For this review, take the finished solid that the model builds, in its own axes (mm). A direction names the side the tool comes from. Coordinates: 2 decimals unless noted, no trailing zeros. Write each loop counter-clockwise with the first axis right and the second up, starting at its lowest first coordinate (ties: lowest second). Pieces come first, ordered by that corner, then holes. Notation, with made-up numbers: (71.5, 4.5) - (116.5, 4.5) arc R17 cw to (116.5, 11.5) - close; hole circle Ø7 at (4, -8.75). An arc over 180 degrees is marked (long way). Use one line per item in the form item = value. Start each with the question number.
1) Mouldability with a two-part tool opening along Y and no side actions: class faces 1 (the flat face through (0, 16.244, 4)), 2 (the flat face through (0, -16.244, 4)), 3 (the flat face through (0, -18.2, 2)), 4 (the flat face through (-5, 21, 2)) as pulls with the +Y half, pulls with the -Y half, needs draft (parallel to the pull), parting line crosses it, or undercut.
2) We need section B-B (y = 15). Give the boundary of the cut face in (x, z).
3) Insertion check: P1, Ø1.5, axis at x = -3, y = 15, coming from the +Z side; P2, Ø3, axis at y = 23.5, z = 4.5, coming from the +X side; P3, Ø1, axis at x = -13, z = 4.5, coming from the +Y side. Each pin has a flat end and moves straight along its axis. Give the tip position at first contact, or say it passes through.
4) We need section A-A (x = 0). Give the boundary of the cut face in (y, z), plus the area to 3 significant figures.
5) We need section C-C (z = 1.95). Give the boundary of the cut face in (x, y).
6) Tool access review of faces 5 (the cylindrical face through (-0.867, 19.295, 3.986)), 6 (the flat face through (-10, 18.2, 2)), 7 (the flat face through (-14, 12.244, 4)): name each direction out of +Z, -Z, +X, -X, +Y, -Y from which nothing blocks a thin tool from reaching the whole face with its end or side.
7) For L1, parallel to Y at x = 0, z = 4.05; L2, parallel to X at y = 14, z = 4.45; L3, parallel to Y at x = 10.5, z = 4.2, list the stretches that pass through material, from the lowest coordinate up. Write a range as from..to.
```python
from build123d import *

# Parameters (mm, degrees)
F1_DEPTH = 3
F0_R     = 4
F2_DEPTH = 5
F3_DEPTH = 2


with BuildPart() as f1:
    # F0 (on Top) → F1 (new body)
    with BuildSketch(Plane.XY):
        Polygon((-12.55, -16.2437940022), (12.55, -16.2437940022), (12.55, 16.2437940022), (-12.55, 16.2437940022), (-12.55, 12.2437940022), (-12.55, 10.2437940022), align=None)
    extrude(amount=F1_DEPTH)



with BuildPart() as f1b:
    # F0 (on Top) → F1, piece 2 (new body)
    with BuildSketch(Plane.XY):
        with Locations((0, 23.1997125853)):
            Circle(F0_R)
    extrude(amount=F1_DEPTH)


with BuildPart() as f1_1:
    add(f1.part)

    add(f1b.part)  # F2 merges F1b
    # F0 (on Top) → F2 (join)
    with BuildSketch(Plane.XY):
        Polygon((12.55, 16.2437940022), (12.55, -16.2437940022), (-12.55, -16.2437940022), (-12.55, 10.2437940022), (-14.55, 10.2437940022), (-14.55, -18.1997125853), (2.482398646, -18.1997125853), (14.55, -18.1997125853), (14.55, 18.1997125853), (5, 18.1997125853), (0, 18.1997125853), (-5, 18.1997125853), (-14.55, 18.1997125853), (-14.55, 12.2437940022), (-12.55, 12.2437940022), (-12.55, 16.2437940022), align=None)
        with BuildLine():
            ThreePointArc((-5, 23.1997125853), (-3.5355339059, 19.6641786794), (0, 18.1997125853))
            ThreePointArc((0, 18.1997125853), (3.5355339059, 19.6641786794), (5, 23.1997125853))
            ThreePointArc((5, 23.1997125853), (0, 28.1997125853), (-5, 23.1997125853))
        make_face()
        with Locations((0, 23.1997125853)):
            Circle(F0_R, mode=Mode.SUBTRACT)
        with BuildLine():
            ThreePointArc((5, 23.1997125853), (3.5355339059, 19.6641786794), (0, 18.1997125853))
            Line((0, 18.1997125853), (5, 18.1997125853))
            Line((5, 18.1997125853), (5, 19.1997125853))
            Line((5, 19.1997125853), (5, 20.1997125853))
            Line((5, 20.1997125853), (5, 23.1997125853))
        make_face()
        with BuildLine():
            Line((-5, 23.1997125853), (-5, 18.1997125853))
            Line((-5, 18.1997125853), (0, 18.1997125853))
            ThreePointArc((0, 18.1997125853), (-3.5355339059, 19.6641786794), (-5, 23.1997125853))
        make_face()
    extrude(amount=F2_DEPTH)

    # F3 (add): a face of the model
    f3_faces = [f1_1.faces().sort_by_distance(p)[0] for p in [
        (-12.55, 11.2437940022, 1.5),
    ]]
    extrude(f3_faces, amount=F3_DEPTH)


solid = f1_1.part
```
Determined:
q1.face_1 = undercut
q1.face_2 = undercut
q1.face_3 = pulls with the -Y half
q1.face_4 = needs draft
q2.outline = (-14.55, 0) - (14.55, 0) - (14.55, 5) - (12.55, 5) - (12.55, 3) - (-12.55, 3) - (-12.55, 5) - (-14.55, 5) - close
q3.P1 = 3
q3.P2 = 5
q3.P3 = 18.2
q4.outline = (-18.2, 0) - (28.2, 0) - (28.2, 5) - (27.2, 5) - (27.2, 3) - (19.2, 3) - (19.2, 5) - (16.24, 5) - (16.24, 3) - (-16.24, 3) - (-16.24, 5) - (-18.2, 5) - close
q4.area = 151 mm²
q5.outline = (-14.55, -18.2) - (14.55, -18.2) - (14.55, 18.2) - (5, 18.2) - (5, 23.2) arc R5 ccw to (-5, 23.2) - (-5, 18.2) - (-14.55, 18.2) - close
q6.face_5 = +Z
q6.face_6 = +Z, -Z, -X, +Y
q6.face_7 = +Z, -X
q7.L1 = -18.2..-16.24, 16.24..19.2, 27.2..28.2
q7.L2 = -14.55..-12.55, 12.55..14.55
q7.L3 = -18.2..-16.24, 16.24..18.2
